Work out the finished part from the listing and answer in its coordinate system (mm). Face numbers are marked on the shaded views. A direction names the side the tool comes from. Coordinates: 2 decimals unless noted, no trailing zeros. Loops run counter-clockwise (first coordinate to the right, second up) from the corner with the lowest first, then second, coordinate; pieces in that order, holes last. Notation, with made-up numbers: (50, 37.25) -> (72, 37.25) arc R19 ccw to (72, 53.25) -> close; hole circle Ø11 at (72, 56.25). An arc over 180 degrees is marked (long way). Use a Markdown table: item, result.
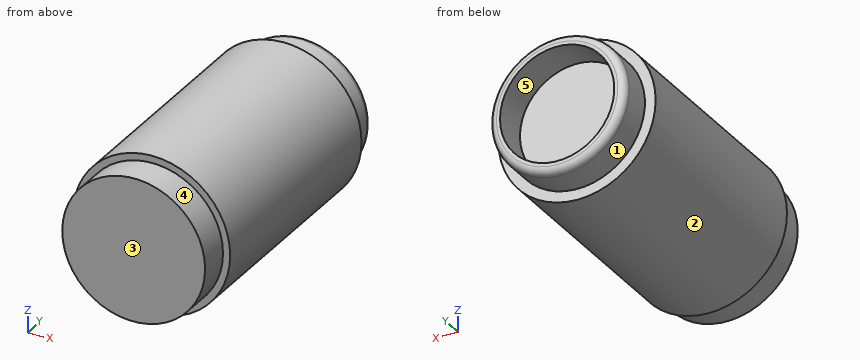
Autodesk Inventor part; units mm, degrees
ref_plane "YZ Plane" through (0, 0, 0) normal (1, 0, 0) x (0, 1, 0)
ref_plane "XZ Plane" through (0, 0, 0) normal (0, 1, 0) x (-1, 0, 0)
ref_plane "XY Plane" through (0, 0, 0) normal (0, 0, 1) x (1, 0, 0)
sketch "Sketch1" plane through (0, 0, 0) normal (0, 1, 0) x (-1, 0, 0)
  circle A0 centre (0, 0) radius 12
  dimension "d0" = 24
extrude "Extrusion1" add sketch "Sketch1" along normal blind 42
sketch "Sketch2" plane through (0, 0, 0) normal (0, -1, 0) x (1, 0, 0)
  circle A0 centre (0, 0) radius 10
  circle A1 centre (0, 0) radius 12
  dimension "d3" = 20
extrude "Extrusion2" cut sketch "Sketch2" against normal blind 4
sketch "Sketch3" plane through (0, 42, 0) normal (0, 1, 0) x (1, 0, 0)
  circle A0 centre (0, 0) radius 9.5
  circle A1 centre (0, 0) radius 12
  dimension "d6" = 19
extrude "Extrusion3" cut sketch "Sketch3" against normal blind 3
move faces "Move1" translate (0, -0.5, 0) faces at (-3.2365, 0, -3.6231)
offset faces "Size1" outward -1 faces at (-11.9611, 15.6667, 0.9656)
move faces "Move2" translate (0, -2, 0) faces at (-10.3014, 39, 1.6353)
sketch "Sketch5" plane through (0, 42, 0) normal (0, 1, 0) x (1, 0, 0)
  circle A0 centre (0, 0) radius 8
  circle A1 centre (0, 0) radius 9.5
  dimension "d20" = 16
extrude "Extrusion5" cut sketch "Sketch5" against normal blind 5 contours A0
fillet "Fillet2" radius 1 1 edges at (-9.5, 42, 0)
properties part number "10x Obj Lens Finite 160mm"
Q1. Section C-C on y = 18 is taken. Determine the outline of the cut face in (x, z), and give its area (3 significant figures).
Solved:
| item | result |
|---|---|
| outline | circle Ø22 at (0, 0) |
| area | 380 mm² |
Q2. Determine the mould class of the marked faces 3, 4 and 5 for opening direction X: pulls with the +X half, pulls with the -X half, needs draft (parallel to the pull), parting line crosses it, or undercut.
Solved:
| item | result |
|---|---|
| face 3 | needs draft |
| face 4 | parting line crosses it |
| face 5 | undercut |
Q3. Consider line 1 (Z direction, x = 0, y = 38.1); line 2 (Y direction, x = 2.5, z = 3). Determine where each line is inside the solid, lowest interval first. Write a range as [from, to].
Solved:
| item | result |
|---|---|
| line 1 | [-9.5, -8], [8, 9.5] |
| line 2 | [-0.5, 37] |
Q4. Section B-B on z = 0 is taken. Determine the outline of the cut face in (x, y), and give its area (3 significant figures).
Solved:
| item | result |
|---|---|
| outline | (-11, 4) -> (-10, 4) -> (-10, -0.5) -> (10, -0.5) -> (10, 4) -> (11, 4) -> (11, 37) -> (9.5, 37) -> (9.5, 41) arc R1 ccw to (8.5, 42) -> (8, 42) -> (8, 37) -> (-8, 37) -> (-8, 42) -> (-8.5, 42) arc R1 ccw to (-9.5, 41) -> (-9.5, 37) -> (-11, 37) -> close |
| area | 831 mm² |
Q5. For the marked faces 1 and 2, determine the directions among +Z, -Z, +X, -X, +Y, -Y from which every point of the face is accessible in a straight line to the end or side of a thin tool.
Solved:
| item | result |
|---|---|
| face 1 | +Y |
| face 2 | +Y, -Y |
Q6. Section A-A on x = 0 is taken. Determine the outline of the cut face in (y, z), and give its area (3 significant figures).
Solved:
| item | result |
|---|---|
| outline | (-0.5, -10) -> (4, -10) -> (4, -11) -> (37, -11) -> (37, -9.5) -> (41, -9.5) arc R1 ccw to (42, -8.5) -> (42, -8) -> (37, -8) -> (37, 8) -> (42, 8) -> (42, 8.5) arc R1 ccw to (41, 9.5) -> (37, 9.5) -> (37, 11) -> (4, 11) -> (4, 10) -> (-0.5, 10) -> close |
| area | 831 mm² |
Q7. Given pin 1 Ø6 at (x, y) = (3.5, 16) entering from -Z; pin 2 Ø2 at (y, z) = (9.5, 6) entering from -X; pin 3 Ø1 at (x, y) = (7, 7.5) entering from +Z, each flat-ended and moving along its own axis, determine where each tip first touches the part or whether it passes through.
Solved:
| item | result |
|---|---|
| pin 1 | z = -10.99 |
| pin 2 | x = -9.8 |
| pin 3 | z = 8.87 |
